Part model, mm, in its own coordinate system. Face numbers are marked on the shaded views. Round coordinates to 2 decimals unless told otherwise and drop trailing zeros. Loops run counter-clockwise (first coordinate to the right, second up) from the corner with the lowest first, then second, coordinate; pieces in that order, holes last. Notation, with made-up numbers: M 59,-5 L 102,-5 A13 ccw 102,19 Z; hole C 51,87.25 d6. An arc over 180 degrees is marked long. Put each result on its own line as item: value. Start each with the question number.
1) Pull direction X, two halves, no side cores. Call the marked faces 1, 2 and 3: +X half, -X half, draft (parallel to the pull), parting line (faces both ways), or undercut.
2) Drop flat-ended pins along their axis: pin 1 Ø20 at (x, y) = (0, 0) entering from +Z; pin 2 Ø1.2 at (y, z) = (-21.5, 34) entering from +X; pin 3 Ø1.5 at (y, z) = (15.5, 28) entering from +X; pin 4 Ø2 at (x, z) = (20, 40.5) entering from -Y. Give the stop position or say it passes through.
3) Slice it at B-B on z = 52. State how many separate pieces and enclosed holes the cut face has, then the cut area to 3 significant figures.
4) Probe line 1 along Y through (x, z) = (0, 47); line 2 along Y through (x, z) = (4, 22.5); line 3 along X through (y, z) = (-3, 5.5). List the from-to ranges inside material, lowest first.
5) Slice it at C-C on y = 13. Give the cut face in (x, z), then the cut area to 3 significant figures.
6) Slice it at A-A on x = 0. Give the cut face in (y, z), then the cut area to 3 significant figures.
```python
from build123d import *

# Parameters (mm, degrees)
F1_R     = 30
F1_R_2   = 16.5
F2_DEPTH = 2.4
F0_R     = 25
F0_R_2   = 16.5
F3_DEPTH = 70
F4_W     = 0.4
F4_H     = 2
F6_R     = 1


with BuildPart() as f2:
    # F1 (on Top) → F2 (new body)
    with BuildSketch(Plane.XY):
        Circle(F1_R)
        Circle(F1_R_2, mode=Mode.SUBTRACT)
    extrude(amount=-F2_DEPTH)

    # F0 (on Top) → F3 (join)
    with BuildSketch(Plane.XY):
        Circle(F0_R)
        with BuildLine():
            ThreePointArc((23.769729, 1.2), (23.792431, 0.600191), (23.8, 0))
            ThreePointArc((23.8, 0), (23.792431, -0.600191), (23.769729, -1.2))
            ThreePointArc((23.769729, -1.2), (16.829141, -16.829141), (1.2, -23.769729))
            ThreePointArc((1.2, -23.769729), (0, -23.8), (-1.2, -23.769729))
            ThreePointArc((-1.2, -23.769729), (-16.829141, -16.829141), (-23.769729, -1.2))
            ThreePointArc((-23.769729, -1.2), (-23.8, 0), (-23.769729, 1.2))
            ThreePointArc((-23.769729, 1.2), (-16.829141, 16.829141), (-1.2, 23.769729))
            ThreePointArc((-1.2, 23.769729), (0, 23.8), (1.2, 23.769729))
            ThreePointArc((1.2, 23.769729), (16.829141, 16.829141), (23.769729, 1.2))
        make_face(mode=Mode.SUBTRACT)
        with BuildLine():
            Line((-17.659275, 1.2), (-23.769729, 1.2))
            ThreePointArc((-23.769729, 1.2), (-23.8, 0), (-23.769729, -1.2))
            Line((-23.769729, -1.2), (-17.659275, -1.2))
            ThreePointArc((-17.659275, -1.2), (-17.7, 0), (-17.659275, 1.2))
        make_face()
        with BuildLine():
            Line((1.2, 17.659275), (1.2, 23.769729))
            ThreePointArc((1.2, 23.769729), (0, 23.8), (-1.2, 23.769729))
            Line((-1.2, 23.769729), (-1.2, 17.659275))
            ThreePointArc((-1.2, 17.659275), (0, 17.7), (1.2, 17.659275))
        make_face()
        with BuildLine():
            ThreePointArc((23.769729, -1.2), (23.792431, -0.600191), (23.8, 0))
            ThreePointArc((23.8, 0), (23.792431, 0.600191), (23.769729, 1.2))
            Line((23.769729, 1.2), (17.659275, 1.2))
            ThreePointArc((17.659275, 1.2), (17.689816, 0.600345), (17.7, 0))
            ThreePointArc((17.7, 0), (17.689816, -0.600345), (17.659275, -1.2))
            Line((17.659275, -1.2), (23.769729, -1.2))
        make_face()
        with BuildLine():
            ThreePointArc((-1.2, -23.769729), (0, -23.8), (1.2, -23.769729))
            Line((1.2, -23.769729), (1.2, -17.659275))
            ThreePointArc((1.2, -17.659275), (0, -17.7), (-1.2, -17.659275))
            Line((-1.2, -17.659275), (-1.2, -23.769729))
        make_face()
        with BuildLine():
            ThreePointArc((17.7, 0), (17.689816, 0.600345), (17.659275, 1.2))
            ThreePointArc((17.659275, 1.2), (12.51579, 12.51579), (1.2, 17.659275))
            ThreePointArc((1.2, 17.659275), (0, 17.7), (-1.2, 17.659275))
            ThreePointArc((-1.2, 17.659275), (-12.51579, 12.51579), (-17.659275, 1.2))
            ThreePointArc((-17.659275, 1.2), (-17.7, 0), (-17.659275, -1.2))
            ThreePointArc((-17.659275, -1.2), (-12.51579, -12.51579), (-1.2, -17.659275))
            ThreePointArc((-1.2, -17.659275), (0, -17.7), (1.2, -17.659275))
            ThreePointArc((1.2, -17.659275), (12.51579, -12.51579), (17.659275, -1.2))
            ThreePointArc((17.659275, -1.2), (17.689816, -0.600345), (17.7, 0))
        make_face()
        Circle(F0_R_2, mode=Mode.SUBTRACT)
    extrude(amount=F3_DEPTH)

    # F4 (on Front) → F5 (revolve, cut)
    with BuildSketch(Plane.XZ):
        with Locations((24.8, 69)):
            Rectangle(F4_W, F4_H)
    revolve(axis=Axis((0, 0, 41.403618), (0, 0, 1)), mode=Mode.SUBTRACT)

    # F6
    f6_edges = [f2.edges().sort_by_distance(p)[0] for p in [
        (-1.2, 23.769729, 35),
        (-1.2, 17.659275, 35),
        (1.2, 23.769729, 35),
        (1.2, 17.659275, 35),
        (17.659275, 1.2, 35),
        (17.659275, -1.2, 35),
        (1.2, -17.659275, 35),
        (-1.2, -17.659275, 35),
        (-17.659275, -1.2, 35),
        (1.2, -23.769729, 35),
        (23.769729, -1.2, 35),
        (23.769729, 1.2, 35),
        (-1.2, -23.769729, 35),
        (-23.769729, -1.2, 35),
        (-23.769729, 1.2, 35),
    ]]
    fillet(f6_edges, radius=F6_R)


solid = f2.part
```
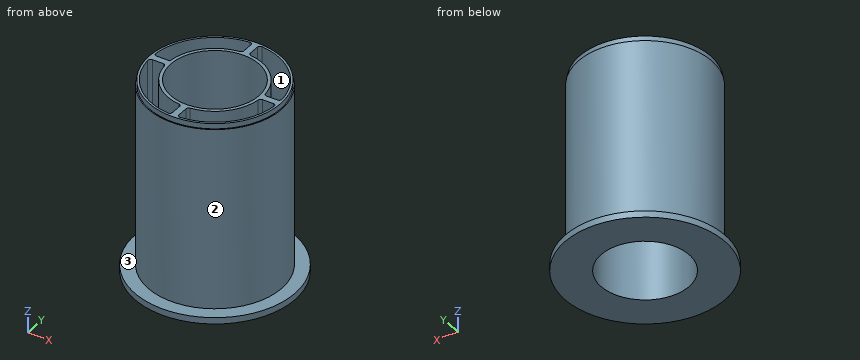
Recorded:
1. face 1: undercut
1. face 2: parting line
1. face 3: draft
2. pin 1: passes through
2. pin 2: stops at x = 13.72
2. pin 3: stops at x = 20.19
2. pin 4: stops at y = -16.25
3. separate pieces: 1
3. enclosed holes: 5
3. area: 375 mm2
4. line 1: y = -25 to -16.5, 16.5 to 25
4. line 2: y = -24.68 to -23.46, -17.24 to -16.01, 16.01 to 17.24, 23.46 to 24.68
4. line 3: x = -24.82 to -23.61, -17.44 to -16.22, 16.22 to 17.44, 23.61 to 24.82
5. outline: M -27.04,-2.4 L -10.16,-2.4 L -10.16,70 L -12.01,70 L -12.01,0 L -19.94,0 L -19.94,70 L -20.88,70 L -20.88,68 L -21.35,68 L -21.35,0 L -27.04,0 Z; M 10.16,-2.4 L 27.04,-2.4 L 27.04,0 L 21.35,0 L 21.35,68 L 20.88,68 L 20.88,70 L 19.94,70 L 19.94,0 L 12.01,0 L 12.01,70 L 10.16,70 Z
5. area: 537 mm2
6. outline: M -30,-2.4 L -16.5,-2.4 L -16.5,70 L -24.6,70 L -24.6,68 L -25,68 L -25,0 L -30,0 Z; M 16.5,-2.4 L 30,-2.4 L 30,0 L 25,0 L 25,68 L 24.6,68 L 24.6,70 L 16.5,70 Z
6. area: 1,250 mm2
